Solid Edge part; units mm, degrees
sketch "Sketch1" plane through (0, 0, 0) normal (0, 0, 1) x (1, 0, 0)
  circle A0 centre (0, 0) radius 1.5
extrude "Protrusion1" add sketch "Sketch1" along normal blind 30
sketch "Sketch2" plane through (0, 0, 30) normal (0, 0, 1) x (1, 0, 0)
  circle A0 centre (0, 0) radius 3
extrude "ExtrudedProtrusion_2" add sketch "Sketch2" along normal blind 1.75
chamfer "Chamfer_1" distance 1.75 angle 45 1 edges at (-3, 0, 30)
sketch "Sketch3" plane through (0, 0, 31.75) normal (0, 0, 1) x (0, 1, 0)
  line L0 (0.8978, -1.555) -> (1.7956, 0)
  line L1 (1.7956, 0) -> (0.8978, 1.555)
  line L2 (0.8978, 1.555) -> (-0.8978, 1.555)
  line L3 (-0.8978, 1.555) -> (-1.7956, 0)
  line L4 (-1.7956, 0) -> (-0.8978, -1.555)
  line L5 (-0.8978, -1.555) -> (0.8978, -1.555)
extrude "ExtrudedCutout_1" cut sketch "Sketch3" against normal blind 1
sketch "Sketch4" plane through (0, 0, 0) normal (0, 0, -1) x (0, 1, 0)
  circle A0 centre (0, 0) radius 1.9215
extrude "ExtrudedCutout_2" cut sketch "Sketch4" against normal blind 21.75
revolve "RevolvedCutout1" [suppressed]
fillet "Round_1" [suppressed]
properties material "Iron, grey cast type 20"
Input: part model. Units: mm. Frame: model coordinates. A direction names the side the tool comes from. Give positions to 0.01 mm unless a question says otherwise; leave off trailing zeros. Loops run counter-clockwise (first coordinate to the right, second up) from the corner with the lowest first, then second, coordinate; pieces in that order, holes last. Notation, with made-up numbers: (-2.75, -24.75) -> (26.25, -24.75) arc R35 ccw to (26.25, 12.25) -> close; hole circle Ø11 at (-0.5, 81). An arc over 180 degrees is marked (long way). Use a Markdown table: item, result.
Q1. Access query for faces 4 (the flat face through (0, 0, 21.75)), 5 (the flat face through (0.77, -1.35, 31.26)). Directions: +Z, -Z, +X, -X, +Y, -Y. A direction counts if a zero-diameter tool reaches every point of the face in a straight line with its end or side. Return the directions, or none.
Entries:
| item | result |
|---|---|
| face 4 | -Z, +X, -X, +Y, -Y |
| face 5 | +Z |
Q2. First-contact query: P1, Ø1, axis at x = 1, z = 26, coming from the +Y side; P2, Ø2, axis at y = 0, z = 29, coming from the -X side; P3, Ø1.6, axis at x = 0.5, y = -0.5, coming from the +Z side. Flat tips, straight axial feed; report the tip coordinate or a pass-through.
Entries:
| item | result |
|---|---|
| P1 | stops at y = 1.41 |
| P2 | stops at x = -1.5 |
| P3 | stops at z = 30.75 |
Q3. Section query B-B, the plane y = 0. Return the cut outline in (x, z) (3 decimals).
Entries:
| item | result |
|---|---|
| outline | (-3, 31.75) -> (-1.5, 30.25) -> (-1.5, 21.75) -> (1.5, 21.75) -> (1.5, 30.25) -> (3, 31.75) -> (1.555, 31.75) -> (1.555, 30.75) -> (-1.555, 30.75) -> (-1.555, 31.75) -> close |
Q4. Pull-direction query (X, two-part tool) for faces 1 (the cylindrical face through (-1.5, -0.07, 25.94)), 2 (the flat face through (0, 0, 30.75)), 3 (the flat face through (1.3, -1.3, 31.75)); classes: pulls with the +X half, pulls with the -X half, needs draft (parallel to the pull), parting line crosses it, or undercut.
Entries:
| item | result |
|---|---|
| face 1 | parting line crosses it |
| face 2 | undercut |
| face 3 | needs draft |
Q5. Section query C-C, the plane z = 27.25. Return the cut outline in (x, y).
Entries:
| item | result |
|---|---|
| outline | circle Ø3 at (0, 0) |
Q6. Section query A-A, the plane z = 31.25. Return the cut outline in (x, y) (3 decimals).
Entries:
| item | result |
|---|---|
| outline | circle Ø5 at (0, 0); hole (-1.555, -0.898) -> (0, -1.796) -> (1.555, -0.898) -> (1.555, 0.898) -> (0, 1.796) -> (-1.555, 0.898) -> close |
Q7. Ray query, probe 1 along Y at (x, z) = (-1.2, 26.25); probe 2 along Z at (x, y) = (0.6, 0.6); probe 3 along X at (y, z) = (-0.1, 28). Return the intervals inside material, ascending. Write a range as from..to.
Entries:
| item | result |
|---|---|
| probe 1 | y = -0.9..0.9 |
| probe 2 | z = 21.75..30.75 |
| probe 3 | x = -1.5..1.5 |
